Autodesk Fusion 360 part; units mm, degrees
sketch "Sketch1" plane through (0, 0, 0) normal (0, 1, 0) x (1, 0, 0)
  line L0 (125, 125) -> (-125, 125) construction
  line L1 (-125, 125) -> (-125, -125) construction
  line L2 (-125, -125) -> (125, -125) construction
  line L3 (125, -125) -> (125, 125) construction
  line L4 (125, 125) -> (-125, -125) construction
  line L5 (-125, 125) -> (125, -125) construction
  line L6 (75, 112.1152) -> (-75, 112.1152) construction
  line L7 (-75, 112.1152) -> (-75, 91.9152) construction
  line L8 (-75, 91.9152) -> (75, 91.9152) construction
  line L9 (75, 91.9152) -> (75, 112.1152) construction
  line L10 (75, 112.1152) -> (-75, 91.9152) construction
  line L11 (-75, 112.1152) -> (75, 91.9152) construction
  line L12 (137, 137) -> (92, 137)
  line L13 (92, 137) -> (137, 92)
  line L14 (137, 92) -> (137, 137)
  line L15 (125, 125) -> (137, 137) construction
  line L16 (128, 128) -> (109, 128) construction
  line L17 (109, 128) -> (128, 109) construction
  line L18 (128, 109) -> (128, 128) construction
  line L19 (92, 137) -> (84, 137)
  line L20 (84, 137) -> (84, 114)
  line L21 (84, 114) -> (104, 114)
  line L22 (104, 114) -> (114, 104)
  line L23 (114, 104) -> (114, 84)
  line L24 (114, 84) -> (137, 84)
  line L25 (137, 84) -> (137, 92)
  line L26 (84, 138) -> (-84, 138)
  line L27 (-84, 138) -> (-84, 113)
  line L28 (-84, 113) -> (84, 113)
  line L29 (84, 113) -> (84, 138)
  line L30 (84, 138) -> (-84, 113) construction
  line L31 (-84, 138) -> (84, 113) construction
  point P0 (0, 102.0152)
  point P1 (0, 125.5)
  dimension "d4" = 250
  dimension "d5" = 250
  dimension "d6" = 150
  dimension "d7" = 20.2
  dimension "d8" = 12
  dimension "d9" = 12
  dimension "d10" = 45
  dimension "d11" = 16
  dimension "d12" = 3
  dimension "d13" = 8
  dimension "d14" = 23
  dimension "d15" = 20
  dimension "d16" = 25
  dimension "d17" = 1
ref_plane "WorkPlane1" through (0, 8, 0) normal (0, 1, 0) x (0, 0, 1)
extrude "Extrude2" add sketch "Sketch1" along normal blind 16.25 contours L13 L19 L20 L21 L22 L23 L24 L25 L29
extrude "Extrude3" add sketch "Sketch1" along normal blind 30 contours L12 L13 L14
sketch "Sketch2" plane through (0, 30, 0) normal (0, 1, 0) x (-1, 0, 0)
  line L0 (-137, -92) -> (-137, -137)
  line L1 (-137, -137) -> (-92, -137)
  line L2 (-92, -137) -> (-137, -92)
  point P0 (-109, -128)
  point P1 (-128, -109)
sketch "Sketch4" plane through (0, 30, 0) normal (0, 1, 0) x (-1, 0, 0)
  line L0 (-137, -92) -> (-137, -137)
  line L1 (-137, -137) -> (-92, -137)
  line L2 (-92, -137) -> (-137, -92)
  point P0 (-128, -128)
  point P1 (-125, -125)
hole "Hole2" at (125, 30, -125) direction (0, -1, 0) diameter 6.2 end through all counterbore diameter 14 counterbore depth 26
sketch "Sketch5" plane through (0, 30, 0) normal (0, 1, 0) x (-1, 0, 0)
  line L0 (-137, -92) -> (-137, -137)
  line L1 (-137, -137) -> (-92, -137)
  line L2 (-92, -137) -> (-137, -92)
  circle A0 centre (-125, -125) radius 7
  point P0 (-109, -128)
  point P1 (-128, -109)
hole "Hole3" at (109, 30, -128) at (128, 30, -109) direction (0, -1, 0) diameter 7.9 depth 13.7 tip angle 180
sketch "Sketch9" plane through (0, 0, 0) normal (0, -1, 0) x (1, 0, 0)
  line L0 (84, -137) -> (137, -137)
  line L1 (137, -137) -> (137, -84)
  line L2 (137, -84) -> (114, -84)
  line L3 (114, -84) -> (114, -104)
  line L4 (114, -104) -> (104, -114)
  line L5 (104, -114) -> (84, -114)
  line L6 (84, -114) -> (84, -137)
  line L7 (84, -119.5) -> (90, -118)
  line L8 (90, -118) -> (90, -133)
  line L9 (90, -133) -> (84, -131.5)
  line L10 (90, -125.5) -> (84, -125.5) construction
  line L11 (84, -119.5) -> (90, -133) construction
  line L12 (84, -131.5) -> (90, -118) construction
  circle A0 centre (125, -125) radius 3.1
  dimension "d51" = 12
  dimension "d52" = 15
  dimension "d53" = 6
extrude "Extrude7" cut sketch "Sketch9" against normal blind 4.4 contours L6 L7 L8 L9
fillet "Fillet1" radius 1 2 edges at (84, 2.2, -119.5) (84, 2.2, -131.5)
fillet "Fillet1" radius 1 2 edges at (90, 2.2, -118) (90, 2.2, -133)
ref_plane "WorkPlane2" through (137, 15, -137) normal (0.7071, 0, 0.7071) x (0, 1, 0)
mirror "Mirror2" about plane through (137, 15, -137) normal (0.7071, 0, 0.7071) of "Extrude7", "Fillet1"
sketch "Sketch10" plane through (0, 16.25, 0) normal (0, 1, 0) x (-1, 0, 0)
  line L0 (-92, -137) -> (-84, -137)
  line L1 (-84, -137) -> (-84, -114)
  line L2 (-84, -114) -> (-104, -114)
  line L3 (-104, -114) -> (-114, -104)
  line L4 (-114, -104) -> (-114, -84)
  line L5 (-114, -84) -> (-137, -84)
  line L6 (-137, -84) -> (-137, -92)
  line L7 (-137, -92) -> (-92, -137)
  line L8 (-84, -134) -> (-134, -84)
extrude "Extrude8" cut sketch "Sketch10" against normal blind 8 contours L1 L2 L8 | L4 L5 L8
fillet "Fillet2" radius 6 1 edges at (137, 15, -137)
fillet "Fillet3" radius 2 2 edges at (92, 23.125, -137) (137, 23.125, -92)
fillet "Fillet4" radius 6 2 edges at (104, 4.125, -114) (114, 4.125, -104)
fillet "Fillet5" radius 1.5 6 edges at (84, 8.125, -137) (84, 12.25, -134) (84, 4.125, -114) (114, 4.125, -84) (134, 12.25, -84) (137, 8.125, -84)
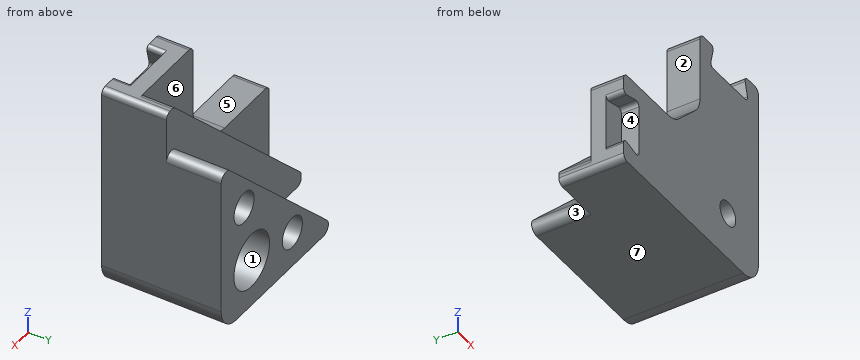
Part model, mm, in its own coordinate system. Face numbers are marked on the shaded views. A direction names the side the tool comes from. Round coordinates to 2 decimals unless told otherwise and drop trailing zeros. Loops run counter-clockwise (first coordinate to the right, second up) from the corner with the lowest first, then second, coordinate; pieces in that order, holes last.
Item 1: Cut at A-A, the plane y = 14.5. Give the cut face in (x, z), then the cut area to 3 significant figures.
Item 2: Cut at B-B, the plane z = -109. Give the cut face in (x, y), then the cut area to 3 significant figures.
Item 3: Mould opens along Z. For the marked faces 1, 2 and 3 say: +Z half, -Z half, draft (parallel to the pull), parting line (faces both ways), or undercut.
Item 4: Drop flat-ended pins along their axis: P1, Ø3.5, axis at x = 125, z = -125, coming from the +Y side; P2, Ø1.5, axis at x = 111, z = -108.5, coming from the +Y side; P3, Ø4, axis at x = 128, z = -111, coming from the +Y side; P4, Ø6.5, axis at y = 6, z = -89.5, coming from the -X side. Give the stop position or say it passes through.
Item 5: Cut at C-C, the plane x = 125. Give the cut face in (y, z), then the cut area to 3 significant figures.
Item 6: Drill centre lines: line 1 (X direction, y = 3.05, z = -125); line 2 (Z direction, x = 128, y = 21.5); line 3 (Z direction, x = 125, y = 2.3). Where is each one in solid material? Low to high.
Item 7: 3-axis set-ups, long thin cutter, end or side, ignore diameter. For the marked faces 4, 5, 6 and 7: which of +Z, -Z, +X, -X, +Y, -Y reach the whole face in a straight line?
Item 8: Cut at D-D, the plane y = 21.75. Give the cut face in (x, z).
A:
1. outline: (84, -135.5) arc R1.5 ccw to (85.5, -137) - (131, -137) arc R6 ccw to (137, -131) - (137, -85.5) arc R1.5 ccw to (135.5, -84) - (134.62, -84) arc R1.5 ccw to (133.56, -84.44) - (84.44, -133.56) arc R1.5 ccw to (84, -134.62) - close; hole circle Ø14 at (125, -125)
1. area: 1,400 mm2
2. outline: (109, 0) - (137, 0) - (137, 30) - (131.95, 30) - (131.95, 16.3) - (124.05, 16.3) - (124.05, 30) - (120, 30) - (120, 16.25) - (109, 16.25) - close
2. area: 581 mm2
3. face 1: undercut
3. face 2: draft
3. face 3: parting line
4. P1: passes through
4. P2: stops at y = 16.25
4. P3: stops at y = 30
4. P4: stops at x = 114
5. outline: (0, -137) - (30, -137) - (30, -132) - (4, -132) - (4, -128.1) - (0, -128.1) - close; (0, -121.9) - (4, -121.9) - (4, -118) - (30, -118) - (30, -111.57) - (16.3, -111.57) - (16.3, -106.43) - (30, -106.43) - (30, -104) - (16.25, -104) - (16.25, -93) - (8.25, -93) - (8.25, -84) - (4.4, -84) - (4.4, -90) - (0, -90) - close
5. area: 757 mm2
6. line 1: x = 90 to 121.9, 128.1 to 137
6. line 2: z = -137 to -131.32, -118.68 to -112.95, -105.05 to -101
6. line 3: z = -137 to -128.1, -121.9 to -90
7. face 4: -X, -Y
7. face 5: +Z, -X, +Y, -Y
7. face 6: +Z, -X, +Y
7. face 7: -Z, +X, -X, +Y, -Y
8. outline: (95.41, -133.59) arc R2 ccw to (96.83, -137) - (131, -137) arc R6 ccw to (137, -131) - (137, -96.83) arc R2 ccw to (133.59, -95.41) - close; hole circle Ø7.9 at (109, -128); hole circle Ø14 at (125, -125); hole circle Ø7.9 at (128, -109)
